Model file for the job. Use its own axes, mm. Face numbers are marked on the shaded views. Round coordinates to 2 decimals unless told otherwise and drop trailing zeros. Order: outer loops, then holes, each group sorted by start corner. A loop starts at its lowest first (then second) coordinate and runs counter-clockwise, first axis right, second up. Notation, with made-up numbers: M -14.5,-13 L 16.5,-13 A18 ccw 16.5,-1 Z; hole C -37,38 d7. An arc over 180 degrees is marked long. Return JSON: item names as keys, results as strings. Group by question number.
Item 1: Probe line 1 along Z through (x, y) = (16.5, 10.25); line 2 along Y through (x, z) = (4, 4.5); line 3 along X through (y, z) = (5.25, 7). List the from-to ranges inside material, lowest first.
Item 2: Slice it at A-A on y = 11. Give the number of separate pieces and of enclosed holes in the cut face, then the cut area to 3 significant figures.
Item 3: Pin check, flat tips, straight feed: pin 1 Ø6 at (x, y) = (-0.5, 2) entering from +Z; pin 2 Ø5 at (y, z) = (6.5, -6) entering from +X; pin 3 Ø12 at (x, z) = (3.5, 3.5) entering from +Y. Stop position of each tip, or through.
Item 4: Slice it at C-C on z = 4. Write the cut outline in (x, y).
Item 5: Pull direction X, two halves, no side cores. Call the marked faces 1 and 2: pulls with the +X half, pulls with the -X half, needs draft (parallel to the pull), parting line crosses it, or undercut.
Item 6: Slice it at B-B on y = 1.25. Write the cut outline in (x, z).
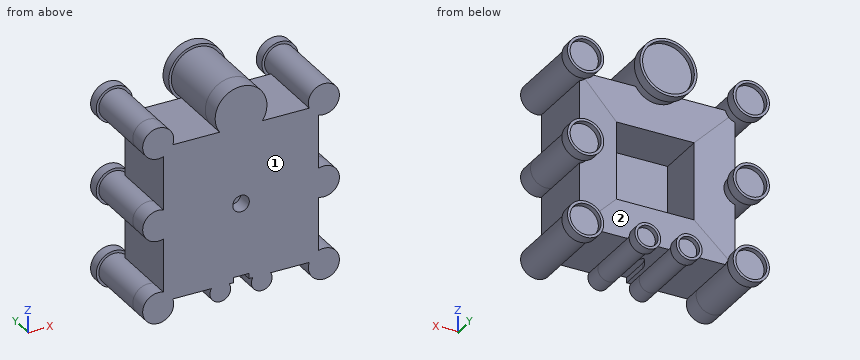
from build123d import *
from build123d.topology import SkipClean

# Parameters (mm, degrees)
CROQUIS1_W              = 30
CROQUIS1_H              = 30
SALIENTE_EXTRUIR1_DEPTH = 10
CROQUIS2_W              = 15
CROQUIS2_H              = 15
CORTAR_EXTRUIR2_DEPTH   = 10
CROQUIS3_W              = 30
CROQUIS3_H              = 30
CORTAR_EXTRUIR3_DEPTH   = 1
CORTAR_EXTRUIR3_DRAFT   = -85
CROQUIS4_R              = 3
CROQUIS4_R_2            = 2
SALIENTE_EXTRUIR3_DEPTH = 12
CROQUIS5_R              = 3.5
CROQUIS5_R_2            = 2.5
SALIENTE_EXTRUIR4_DEPTH = 2
CORTAR_EXTRUIR4_START   = -1
CROQUIS6_R              = 3
CROQUIS6_R_2            = 2
CORTAR_EXTRUIR4_DEPTH   = 1
CORTAR_EXTRUIR5_DEPTH   = 1
SALIENTE_EXTRUIR5_START = 3.5
SALIENTE_EXTRUIR5_DEPTH = 3.5
SALIENTE_EXTRUIR6_REACH = 32.927
CROQUIS9_R              = 5
CROQUIS10_R             = 5.5
SALIENTE_EXTRUIR7_DEPTH = 2
CORTAR_EXTRUIR7_START   = -1
CROQUIS11_R             = 5
CORTAR_EXTRUIR7_DEPTH   = 1
SALIENTE_EXTRUIR8_START = 3.5
SALIENTE_EXTRUIR8_DEPTH = 3.5
CROQUIS13_R             = 1.6
CORTAR_EXTRUIR8_DEPTH   = 3


with BuildPart() as part:
    # Croquis1 → Saliente-Extruir1 (new body)
    with BuildSketch(Plane(origin=(0, 0, 0), x_dir=(1, 0, 0), z_dir=(0, 1, 0))):
        Rectangle(CROQUIS1_W, CROQUIS1_H)
    extrude(amount=SALIENTE_EXTRUIR1_DEPTH)

    # Croquis2 → Cortar-Extruir2 (cut)
    with BuildSketch(Plane(origin=(0, 10, 0), x_dir=(1, 0, 0), z_dir=(0, 1, 0))):
        Rectangle(CROQUIS2_W, CROQUIS2_H)
    extrude(amount=-CORTAR_EXTRUIR2_DEPTH, mode=Mode.SUBTRACT)


with BuildPart() as cortar_extruir3_tool:
    # Croquis3 → Cortar-Extruir3 (with draft: the straight prism first)
    with BuildSketch(Plane(origin=(0, 10, 0), x_dir=(1, 0, 0), z_dir=(0, 1, 0))):
        Rectangle(CROQUIS3_W, CROQUIS3_H)
    extrude(amount=-CORTAR_EXTRUIR3_DEPTH)
    # Cortar-Extruir3: the draft: its side faces are tilted about the plane it starts from
    cortar_extruir3_sides = [cortar_extruir3_tool.faces().sort_by_distance(p)[0] for p in [
        (15, 9.5, 0),
        (0, 9.5, -15),
        (-15, 9.5, 0),
        (0, 9.5, 15),
    ]]
    draft(cortar_extruir3_sides, Plane(origin=(0, 10, 0), x_dir=(1, 0, 0), z_dir=(0, 1, 0)), CORTAR_EXTRUIR3_DRAFT)


with BuildPart() as part_1:
    add(part.part)

    # Cortar-Extruir3: cut by cortar_extruir3_tool
    add(cortar_extruir3_tool.part, mode=Mode.SUBTRACT)

    # Croquis4 → Saliente-Extruir3 (add)
    with BuildSketch(Plane(origin=(0, 0, 0), x_dir=(1, 0, 0), z_dir=(0, 1, 0))):
        with Locations(Location((-16, 16, 0), (0, 0, 340.528779366))):
            Circle(CROQUIS4_R)
        with Locations(Location((16, 16, 0), (0, 0, 199.471220634))):
            Circle(CROQUIS4_R)
        with Locations(Location((16, 0, 0), (0, 0, 109.471220634))):
            Circle(CROQUIS4_R)
        with Locations(Location((16, -16, 0), (0, 0, 109.471220634))):
            Circle(CROQUIS4_R)
        with Locations(Location((-16, 0, 0), (0, 0, 70.528779366))):
            Circle(CROQUIS4_R)
        with Locations(Location((-16, -16, 0), (0, 0, 70.528779366))):
            Circle(CROQUIS4_R)
        with Locations(Location((-4, 16, 0), (0, 0, 330))):
            Circle(CROQUIS4_R_2)
        with Locations(Location((4, 16, 0), (0, 0, 330))):
            Circle(CROQUIS4_R_2)
    extrude(amount=SALIENTE_EXTRUIR3_DEPTH)

    # Croquis5 → Saliente-Extruir4 (add)
    with BuildSketch(Plane(origin=(0, 12, 0), x_dir=(1, 0, 0), z_dir=(0, 1, 0))):
        with Locations(Location((-16, 16, 0), (0, 0, 270))):
            Circle(CROQUIS5_R)
        with Locations(Location((-4, 16, 0), (0, 0, 270))):
            Circle(CROQUIS5_R_2)
        with Locations(Location((4, 16, 0), (0, 0, 270))):
            Circle(CROQUIS5_R_2)
        with Locations(Location((16, 16, 0), (0, 0, 270))):
            Circle(CROQUIS5_R)
        with Locations(Location((-16, 0, 0), (0, 0, 270))):
            Circle(CROQUIS5_R)
        with Locations(Location((16, 0, 0), (0, 0, 270))):
            Circle(CROQUIS5_R)
        with Locations(Location((16, -16, 0), (0, 0, 270))):
            Circle(CROQUIS5_R)
        with Locations(Location((-16, -16, 0), (0, 0, 270))):
            Circle(CROQUIS5_R)
    extrude(amount=SALIENTE_EXTRUIR4_DEPTH)

    # Croquis6 → Cortar-Extruir4 (cut)
    with BuildSketch(Plane(origin=(0, 14, 0), x_dir=(1, 0, 0), z_dir=(0, 1, 0)).offset(CORTAR_EXTRUIR4_START)):
        with Locations(Location((-16, -16, 0), (0, 0, 70.528779366))):
            Circle(CROQUIS6_R)
        with Locations(Location((-16, 0, 0), (0, 0, 70.528779366))):
            Circle(CROQUIS6_R)
        with Locations(Location((-16, 16, 0), (0, 0, 340.528779366))):
            Circle(CROQUIS6_R)
        with Locations(Location((-4, 16, 0), (0, 0, 330))):
            Circle(CROQUIS6_R_2)
        with Locations(Location((4, 16, 0), (0, 0, 330))):
            Circle(CROQUIS6_R_2)
        with Locations(Location((16, 16, 0), (0, 0, 199.471220634))):
            Circle(CROQUIS6_R)
        with Locations(Location((16, 0, 0), (0, 0, 109.471220634))):
            Circle(CROQUIS6_R)
        with Locations(Location((16, -16, 0), (0, 0, 109.471220634))):
            Circle(CROQUIS6_R)
    extrude(amount=CORTAR_EXTRUIR4_DEPTH, mode=Mode.SUBTRACT)

    # Croquis7 → Cortar-Extruir5 (cut)
    with BuildSketch(Plane(origin=(0, 0, -15), x_dir=(-1, 0, 0), z_dir=(0, 0, -1))):
        with BuildLine():
            Line((-1.5, 0), (-1.5, 2))
            add(Edge.make_bspline(
                [(-1.5, 2), (-1.5, 3.25), (0, 5.335598169)],
                knots=[0, 0, 0, 1, 1, 1], degree=2))
            add(Edge.make_bspline(
                [(1.5, 2), (1.5, 3.25), (0, 5.335598169)],
                knots=[0, 0, 0, 1, 1, 1], degree=2))
            Line((1.5, 2), (1.5, 0))
            Line((1.5, 0), (-1.5, 0))
        make_face()
    extrude(amount=-CORTAR_EXTRUIR5_DEPTH, mode=Mode.SUBTRACT)

    # Croquis8 → Saliente-Extruir5 (add)
    with SkipClean():  # the faces are left unmerged after this step: merging them gives an invalid solid
        with BuildSketch(Plane.XZ.offset(SALIENTE_EXTRUIR5_START)):
            with BuildLine():
                Line((-1.5, -15), (-1.5, -14))
                Line((-1.5, -14), (1.5, -14))
                Line((1.5, -14), (1.5, -15))
                Line((1.5, -15), (2.267949192, -15))
                ThreePointArc((2.267949192, -15), (4, -18), (5.732050808, -15))
                Line((5.732050808, -15), (13.171572875, -15))
                ThreePointArc((13.171572875, -15), (18.121320344, -18.121320344), (15, -13.171572875))
                Line((15, -13.171572875), (15, -2.828427125))
                ThreePointArc((15, -2.828427125), (19, 0), (15, 2.828427125))
                Line((15, 2.828427125), (15, 13.171572875))
                ThreePointArc((15, 13.171572875), (18.121320344, 18.121320344), (13.171572875, 15))
                Line((13.171572875, 15), (-13.171572875, 15))
                ThreePointArc((-13.171572875, 15), (-18.121320344, 18.121320344), (-15, 13.171572875))
                Line((-15, 13.171572875), (-15, 2.828427125))
                ThreePointArc((-15, 2.828427125), (-19, 0), (-15, -2.828427125))
                Line((-15, -2.828427125), (-15, -13.171572875))
                ThreePointArc((-15, -13.171572875), (-18.121320344, -18.121320344), (-13.171572875, -15))
                Line((-13.171572875, -15), (-5.732050808, -15))
                ThreePointArc((-5.732050808, -15), (-4, -18), (-2.267949192, -15))
                Line((-2.267949192, -15), (-1.5, -15))
            make_face()
        extrude(amount=-SALIENTE_EXTRUIR5_DEPTH)

    # Saliente-Extruir6: up to this face of the body (flat: up to its plane)
    saliente_extruir6_end = Plane(part_1.part.faces().sort_by_distance((-16, 12, 12.598994949))[0])
    # Croquis9 → Saliente-Extruir6 (add, up to the picked face)
    with BuildSketch(Plane(origin=(0, 0, 0), x_dir=(1, 0, 0), z_dir=(0, 1, 0)), mode=Mode.PRIVATE) as saliente_extruir6_sk1:
        with Locations(Location((0, -17.806013585, 0), (0, 0, 34.139014511))):
            Circle(CROQUIS9_R)
    saliente_extruir6_tool1 = split(extrude(saliente_extruir6_sk1.sketch, amount=SALIENTE_EXTRUIR6_REACH, mode=Mode.PRIVATE), bisect_by=saliente_extruir6_end, keep=Keep.BOTH, mode=Mode.PRIVATE)
    add(saliente_extruir6_tool1.solids().sort_by(Axis((0, 0, 17.806014), (0, 1, 0)))[0])

    # Croquis10 → Saliente-Extruir7 (add)
    with SkipClean():  # the faces are left unmerged after this step: merging them gives an invalid solid
        with BuildSketch(Plane(origin=(0, 12, 0), x_dir=(1, 0, 0), z_dir=(0, 1, 0))):
            with Locations(Location((0, -17.806013585, 0), (0, 0, 270))):
                Circle(CROQUIS10_R)
        extrude(amount=SALIENTE_EXTRUIR7_DEPTH)

    # Croquis11 → Cortar-Extruir7 (cut)
    with SkipClean():  # the faces are left unmerged after this step: merging them gives an invalid solid
        with BuildSketch(Plane(origin=(0, 14, 0), x_dir=(1, 0, 0), z_dir=(0, 1, 0)).offset(CORTAR_EXTRUIR7_START)):
            with Locations(Location((0, -17.806013585, 0), (0, 0, 34.139014511))):
                Circle(CROQUIS11_R)
        extrude(amount=CORTAR_EXTRUIR7_DEPTH, mode=Mode.SUBTRACT)

    # Croquis12 → Saliente-Extruir8 (add)
    with SkipClean():  # the faces are left unmerged after this step: merging them gives an invalid solid
        with BuildSketch(Plane.XZ.offset(SALIENTE_EXTRUIR8_START)):
            with BuildLine():
                Line((-4.138391929, 15), (4.138391929, 15))
                ThreePointArc((4.138391929, 15), (0, 22.806013585), (-4.138391929, 15))
            make_face()
        extrude(amount=-SALIENTE_EXTRUIR8_DEPTH)

    # Croquis13 → Cortar-Extruir8 (cut)
    with SkipClean():  # the faces are left unmerged after this step: merging them gives an invalid solid
        with BuildSketch(Plane.XZ.offset(3.5)):
            with Locations(Location((0, 0, 0), (0, 0, 270))):
                Circle(CROQUIS13_R)
        extrude(amount=-CORTAR_EXTRUIR8_DEPTH, mode=Mode.SUBTRACT)


solid = part_1.part
Output values:
{
 "1": {"line 1": "-18.96 to -13.04, -2.96 to 2.96, 13.04 to 18.96", "line 2": "-3.5 to 0", "line 3": "-15 to -7.5, 7.5 to 15"},
 "2": {"separate pieces": "9", "enclosed holes": "0", "area": "273 mm²"},
 "3": {"pin 1": "z = 22.81", "pin 2": "x = 15", "pin 3": "y = 9.52"},
 "4": {"outline": "M -15,-3.5 L 15,-3.5 L 15,10 L 7.5,9.34 L 7.5,0 L -7.5,0 L -7.5,9.34 L -15,10 Z"},
 "5": {"face 1": "needs draft", "face 2": "undercut"},
 "6": {"outline": "M -15,-13.17 A3 ccw long -13.17,-15 L -5.73,-15 A2 ccw long -2.27,-15 L -1.5,-15 L -1.5,-14 L 1.5,-14 L 1.5,-15 L 2.27,-15 A2 ccw long 5.73,-15 L 13.17,-15 A3 ccw long 15,-13.17 L 15,-2.83 A3 ccw long 15,2.83 L 15,13.17 A3 ccw long 13.17,15 L 4.14,15 A5 ccw long -4.14,15 L -13.17,15 A3 ccw long -15,13.17 L -15,2.83 A3 ccw long -15,-2.83 Z; hole M -7.5,-7.5 L 7.5,-7.5 L 7.5,7.5 L -7.5,7.5 Z"}
}
